Could you check a few things on this model? Use its own coordinates, in mm. A direction names the side the tool comes from. Coordinates: 2 decimals unless noted, no trailing zeros. Loops run counter-clockwise (first coordinate to the right, second up) from the corner with the lowest first, then second, coordinate; pieces in that order, holes last.
1) Thinking about a two-plate mould opening in X: for faces 4 (the face through (-27.36, 12.62, -62.77)), 5 (the face through (-1, 0, -1)), 6 (the face through (24.488, 45.172, -62.774)), which applies, released by +X, released by -X, zero draft, split by the parting line, or undercut?
2) For faces 1 (the face through (-1, 31, 62)), 2 (the face through (-22.854, 13.197, -62.325)), 3 (the face through (83.472, 1.479, -9.834)), which set-ups out of +Z, -Z, +X, -X, +Y, -Y let a thin tool reach every point of the face, with its end or its side?
3) If I drill on line 1 along Z through (x, y) = (77.5, 20.5); line 2 along X through (y, z) = (1.1, -43.5); line 3 along Y through (x, z) = (-25, -62.5), over which ranges is the centre line in solid material (lowest first)?
4) Imagine slicing it at D-D on x = 84.75. Please give me the cut outline in (y, z), plus the area to 3 significant figures.
5) Will these pins go through, and if not, where does the flat tip stop? P1, Ø6.5, axis at x = 74.75, z = -11.5, coming from the +Y side; P2, Ø2.5, axis at x = -74.75, z = 16.5, coming from the -Y side; P3, Ø2.5, axis at x = -25, y = 47.48, coming from the -Z side.
6) Imagine slicing it at A-A on x = -25. Please give me the cut outline in (y, z), plus the area to 3 significant figures.
7) Imagine slicing it at C-C on x = 0. Please give me the cut outline in (y, z).
8) Imagine slicing it at B-B on z = 48.5. Please give me the cut outline in (x, y), plus the area to 3 significant figures.
```python
from build123d import *

# Parameters (mm, degrees)
SKETCH1_W                                            = 188
SKETCH1_H                                            = 130
BOSS_EXTRUDE1_DEPTH                                  = 3
EDGE_FLANGE1_STRIP_W                                 = 20
EDGE_FLANGE1_STRIP_H                                 = 3
EDGE_FLANGE1_STRIP_CUT_DEPTH                         = 188
EDGE_FLANGE1_STRIP_2_W                               = 20
EDGE_FLANGE1_STRIP_2_H                               = 3
EDGE_FLANGE1_STRIP_CUT_2_DEPTH                       = 188
EDGE_FLANGE1_DEPTH                                   = 188
EDGE_FLANGE1_BEND_DEPTH                              = 188
SKETCH8_R                                            = 15
CUT_EXTRUDE1_DEPTH                                   = 10
CSK_FOR_M4_HEX_SOCKET_COUNTERSUNK_HEAD_S_D           = 4.5
CSK_FOR_M4_HEX_SOCKET_COUNTERSUNK_HEAD_S_DEPTH       = 10
CSK_FOR_M4_HEX_SOCKET_COUNTERSUNK_HEAD_S_CSINK_D     = 9.18
CSK_FOR_M4_HEX_SOCKET_COUNTERSUNK_HEAD_S_CSINK_ANGLE = 90
CSK_FOR_M4_HEX_SOCKET_COUNTERSUNK_HEAD_S_TIP         = 1.351936393
SKETCH12_R                                           = 2.1
CUT_EXTRUDE2_DEPTH                                   = 10


# Sheet-metal steps are written as plain solids
with BuildPart() as part:
    # Sketch1 → Boss-Extrude1 (new body)
    with BuildSketch(Plane(origin=(0, 0, 0), x_dir=(1, 0, 0), z_dir=(0, 1, 0))):
        Rectangle(SKETCH1_W, SKETCH1_H)
    extrude(amount=BOSS_EXTRUDE1_DEPTH)

    # Edge-Flange1 strip (across the edge) → Edge-Flange1 strip cut (cut)
    with BuildSketch(Plane(origin=(94, 3, -65), x_dir=(0, 0, 1), z_dir=(-1, 0, 0))):
        with Locations((-3, -1.5)):
            Rectangle(EDGE_FLANGE1_STRIP_W, EDGE_FLANGE1_STRIP_H)
    extrude(amount=EDGE_FLANGE1_STRIP_CUT_DEPTH, mode=Mode.SUBTRACT)

    # Edge-Flange1 strip 2 (across the edge) → Edge-Flange1 strip cut 2 (cut)
    with BuildSketch(Plane(origin=(-94, 3, 65), x_dir=(0, 0, -1), z_dir=(1, 0, 0))):
        with Locations((-3, -1.5)):
            Rectangle(EDGE_FLANGE1_STRIP_2_W, EDGE_FLANGE1_STRIP_2_H)
    extrude(amount=EDGE_FLANGE1_STRIP_CUT_2_DEPTH, mode=Mode.SUBTRACT)

    # Edge-Flange1 section (across the edge) → Edge-Flange1 (add)
    with BuildSketch(Plane(origin=(94, 3, -65), x_dir=(0, 0, 1), z_dir=(-1, 0, 0))):
        with BuildLine():
            Line((0, 4), (0, 52))
            Line((0, 52), (3, 52))
            Line((3, 52), (3, 4))
            ThreePointArc((3, 4), (4.171572875, 1.171572875), (7, 0))
            Line((7, 0), (7, -3))
            ThreePointArc((7, -3), (2.050252532, -0.949747468), (0, 4))
        make_face()
    extrude(amount=EDGE_FLANGE1_DEPTH)

    # Edge-Flange1 section 2 (across the edge) → Edge-Flange1 bend (add)
    with BuildSketch(Plane(origin=(-94, 3, 65), x_dir=(0, 0, -1), z_dir=(1, 0, 0))):
        with BuildLine():
            Line((0, 4), (0, 52))
            Line((0, 52), (3, 52))
            Line((3, 52), (3, 4))
            ThreePointArc((3, 4), (4.171572875, 1.171572875), (7, 0))
            Line((7, 0), (7, -3))
            ThreePointArc((7, -3), (2.050252532, -0.949747468), (0, 4))
        make_face()
    extrude(amount=EDGE_FLANGE1_BEND_DEPTH)

    # Sketch8 → Cut-Extrude1 (cut)
    with BuildSketch(Plane(origin=(0, 0, -65), x_dir=(-1, 0, 0), z_dir=(0, 0, -1))):
        with Locations(Location((0, 30, 0), (0, 0, 90))):
            Circle(SKETCH8_R)
    extrude(amount=-CUT_EXTRUDE1_DEPTH, mode=Mode.SUBTRACT)

    # CSK for M4 Hex Socket Countersunk Head Screw1
    with Locations(Plane(origin=(0, 0, -65), x_dir=(-1, 0, 0), z_dir=(0, 0, -1))):
        with Locations((-25, 47.478966411), (-25, 12.521033589), (25, 47.478966411), (25, 12.521033589)):
            CounterSinkHole(CSK_FOR_M4_HEX_SOCKET_COUNTERSUNK_HEAD_S_D / 2, CSK_FOR_M4_HEX_SOCKET_COUNTERSUNK_HEAD_S_CSINK_D / 2, depth=CSK_FOR_M4_HEX_SOCKET_COUNTERSUNK_HEAD_S_DEPTH, counter_sink_angle=CSK_FOR_M4_HEX_SOCKET_COUNTERSUNK_HEAD_S_CSINK_ANGLE)
            with Locations((0, 0, -(CSK_FOR_M4_HEX_SOCKET_COUNTERSUNK_HEAD_S_DEPTH + CSK_FOR_M4_HEX_SOCKET_COUNTERSUNK_HEAD_S_TIP / 2))):  # 118° drill point
                Cone(0, CSK_FOR_M4_HEX_SOCKET_COUNTERSUNK_HEAD_S_D / 2, CSK_FOR_M4_HEX_SOCKET_COUNTERSUNK_HEAD_S_TIP, mode=Mode.SUBTRACT)

    # Sketch12 → Cut-Extrude2 (cut)
    with BuildSketch(Plane(origin=(0, 0, 0), x_dir=(-1, 0, 0), z_dir=(0, -1, 0))):
        with Locations(Location((74.75, 43.5, 0), (0, 0, 90))):
            Circle(SKETCH12_R)
        with Locations(Location((84.75, 43.5, 0), (0, 0, 90))):
            Circle(SKETCH12_R)
        with Locations(Location((74.75, -16.5, 0), (0, 0, 90))):
            Circle(SKETCH12_R)
        with Locations(Location((84.75, -16.5, 0), (0, 0, 90))):
            Circle(SKETCH12_R)
        with Locations(Location((-74.75, 11.5, 0), (0, 0, 90))):
            Circle(SKETCH12_R)
        with Locations(Location((-84.75, 11.5, 0), (0, 0, 90))):
            Circle(SKETCH12_R)
        with Locations(Location((-74.75, -48.5, 0), (0, 0, 90))):
            Circle(SKETCH12_R)
        with Locations(Location((-84.75, -48.5, 0), (0, 0, 90))):
            Circle(SKETCH12_R)
    extrude(amount=-CUT_EXTRUDE2_DEPTH, mode=Mode.SUBTRACT)


solid = part.part
```
Filled in:
1. face 4: undercut
1. face 5: zero draft
1. face 6: undercut
2. face 1: +X, -X, +Y
2. face 2: -Z
2. face 3: +Y, -Y
3. line 1: z = -65 to -62, 62 to 65
3. line 2: x = -94 to -86.85, -82.65 to -76.85, -72.65 to 94
3. line 3: y = 1.64 to 10.27, 14.77 to 45.23, 49.73 to 55
4. outline: (0, -58) arc R7 ccw to (7, -65) - (55, -65) - (55, -62) - (7, -62) arc R4 cw to (3, -58) - (3, -13.6) - (0, -13.6) - close; (0, -9.4) - (3, -9.4) - (3, 46.4) - (0, 46.4) - close; (0, 50.6) - (3, 50.6) - (3, 58) arc R4 cw to (7, 62) - (55, 62) - (55, 65) - (7, 65) arc R7 ccw to (0, 58) - close
4. area: 663 mm2
5. P1: stops at y = 3
5. P2: passes through
5. P3: stops at z = 62
6. outline: (0, -58) arc R7 ccw to (7, -65) - (7.93, -65) - (10.27, -62.66) - (10.27, -62) - (7, -62) arc R4 cw to (3, -58) - (3, 58) arc R4 cw to (7, 62) - (55, 62) - (55, 65) - (7, 65) arc R7 ccw to (0, 58) - close; (14.77, -62.66) - (17.11, -65) - (42.89, -65) - (45.23, -62.66) - (45.23, -62) - (14.77, -62) - close; (49.73, -62.66) - (52.07, -65) - (55, -65) - (55, -62) - (49.73, -62) - close
6. area: 650 mm2
7. outline: (0, -58) arc R7 ccw to (7, -65) - (15, -65) - (15, -62) - (7, -62) arc R4 cw to (3, -58) - (3, 58) arc R4 cw to (7, 62) - (55, 62) - (55, 65) - (7, 65) arc R7 ccw to (0, 58) - close; (45, -65) - (55, -65) - (55, -62) - (45, -62) - close
8. outline: (-94, 0) - (72.65, 0) - (72.65, 3) - (-94, 3) - close; (76.85, 0) - (82.65, 0) - (82.65, 3) - (76.85, 3) - close; (86.85, 0) - (94, 0) - (94, 3) - (86.85, 3) - close
8. area: 539 mm2
